```python
from build123d import *

# Parameters (mm, degrees)
F0_R     = 1.5875
F1_DEPTH = 3.048


with BuildPart() as f1:
    # F0 (on Front) → F1 (new body)
    with BuildSketch(Plane.XZ):
        with BuildLine():
            ThreePointArc((1.5875, 0), (1.122532, 1.122532), (0, 1.5875))
            ThreePointArc((0, 1.5875), (-1.122532, -1.122532), (1.5875, 0))
        make_face()
        with BuildLine():
            ThreePointArc((0.677344, -9.500886), (6.970557, -6.491299), (9.525, 0))
            ThreePointArc((9.525, 0), (6.735192, 6.735192), (0, 9.525))
            ThreePointArc((0, 9.525), (-6.534492, 6.930082), (-9.50857, 0.559208))
            ThreePointArc((-9.50857, 0.559208), (-6.930082, -6.534492), (0, -9.525))
            Line((0, -9.525), (0.677344, -9.500886))
        make_face()
        with BuildLine():
            ThreePointArc((1.5875, 0), (-1.122532, -1.122532), (0, 1.5875))
            ThreePointArc((0, 1.5875), (1.122532, 1.122532), (1.5875, 0))
        make_face(mode=Mode.SUBTRACT)
        with BuildLine():
            ThreePointArc((0, 9.525), (6.735192, 6.735192), (9.525, 0))
            ThreePointArc((9.525, 0), (6.970557, -6.491299), (0.677344, -9.500886))
            Line((0.677344, -9.500886), (44.732405, -7.932475))
            ThreePointArc((44.732405, -7.932475), (36.513756, -0.141225), (44.45, 7.9375))
            Line((44.45, 7.9375), (18.817909, 8.852932))
            ThreePointArc((18.817909, 8.852932), (13.12642, 11.553818), (11.18688, 17.547649))
            Line((11.18688, 17.547649), (15.064665, 58.492855))
            ThreePointArc((15.064665, 58.492855), (9.28782, 50.625528), (0, 47.625))
            Line((0, 47.625), (0, 9.525))
        make_face()
        with BuildLine():
            ThreePointArc((-9.50857, 0.559208), (-6.534492, 6.930082), (0, 9.525))
            Line((0, 9.525), (0, 47.625))
            ThreePointArc((0, 47.625), (-9.835501, 51.038918), (-15.440753, 59.812348))
            Line((-15.440753, 59.812348), (-9.50857, 0.559208))
        make_face()
        with BuildLine():
            ThreePointArc((0, -9.525), (0.338886, -9.51897), (0.677344, -9.500886))
            Line((0.677344, -9.500886), (0, -9.525))
        make_face()
        with BuildLine():
            Line((0, 61.9125), (0, 47.625))
            ThreePointArc((0, 47.625), (9.28782, 50.625528), (15.064665, 58.492855))
            ThreePointArc((15.064665, 58.492855), (15.671107, 60.963854), (15.875, 63.5))
            ThreePointArc((15.875, 63.5), (15.613359, 66.370305), (14.83706, 69.145998))
            ThreePointArc((14.83706, 69.145998), (9.0107, 76.569924), (0, 79.375))
            Line((0, 79.375), (0, 65.0875))
            ThreePointArc((0, 65.0875), (1.122532, 64.622532), (1.5875, 63.5))
            ThreePointArc((1.5875, 63.5), (1.122532, 62.377468), (0, 61.9125))
        make_face()
        with BuildLine():
            ThreePointArc((-15.440753, 59.812348), (-9.835501, 51.038918), (0, 47.625))
            Line((0, 47.625), (0, 61.9125))
            ThreePointArc((0, 61.9125), (-1.5875, 63.5), (0, 65.0875))
            Line((0, 65.0875), (0, 79.375))
            ThreePointArc((0, 79.375), (-9.835501, 75.961082), (-15.440753, 67.187652))
            ThreePointArc((-15.440753, 67.187652), (-15.875, 63.5), (-15.440753, 59.812348))
        make_face()
        with BuildLine():
            ThreePointArc((44.45, 7.9375), (36.513756, -0.141225), (44.732405, -7.932475))
            ThreePointArc((44.732405, -7.932475), (50.161633, -5.51191), (52.3875, 0))
            ThreePointArc((52.3875, 0), (50.06266, 5.61266), (44.45, 7.9375))
        make_face()
        with Locations((44.45, 0)):
            Circle(F0_R, mode=Mode.SUBTRACT)
        with BuildLine():
            Line((-9.452585, 115.472291), (-15.440753, 67.187652))
            ThreePointArc((-15.440753, 67.187652), (-9.835501, 75.961082), (0, 79.375))
            ThreePointArc((0, 79.375), (9.0107, 76.569924), (14.83706, 69.145998))
            Line((14.83706, 69.145998), (9.461313, 115.399625))
            ThreePointArc((9.461313, 115.399625), (9.509065, 114.850734), (9.525, 114.3))
            ThreePointArc((9.525, 114.3), (-0.587263, 104.793121), (-9.452585, 115.472291))
        make_face()
        with Locations((-2.690725, 100.0252)):
            Circle(F0_R, mode=Mode.SUBTRACT)
        with BuildLine():
            ThreePointArc((9.461313, 115.399625), (0.036594, 123.82493), (-9.452585, 115.472291))
            ThreePointArc((-9.452585, 115.472291), (-0.587263, 104.793121), (9.525, 114.3))
            ThreePointArc((9.525, 114.3), (9.509065, 114.850734), (9.461313, 115.399625))
        make_face()
        with Locations((0.111441, 114.374639)):
            Circle(F0_R, mode=Mode.SUBTRACT)
    extrude(amount=F1_DEPTH)


solid = f1.part
```
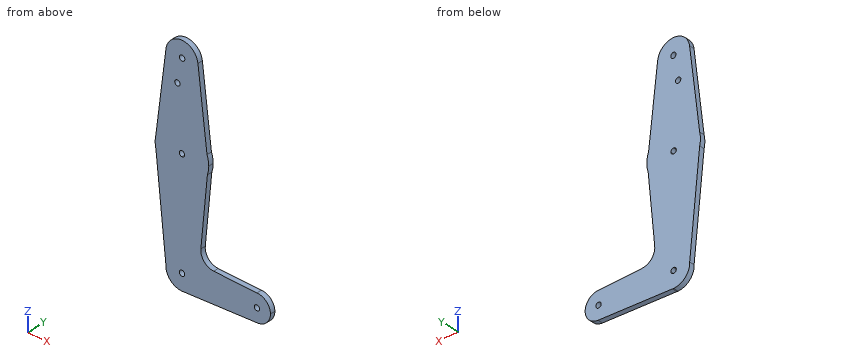
Check sheet for the modelled part. Datum: model origin and axes. Units: mm. Coordinates: 2 decimals unless noted, no trailing zeros. Write each loop counter-clockwise with the first axis right and the second up, starting at its lowest first coordinate (ties: lowest second). Pieces come first, ordered by that corner, then holes. Notation, with made-up numbers: M 14.25,52 L 19.25,52 A20 cw 19.25,74 Z; hole C -38,24.25 d3. An arc over 180 degrees is marked long. Write item = value, one per line. Start each with the question number.
1. Thickness scan on probe 1 along Z at (x, y) = (45, -0.9); probe 2 along Z at (x, y) = (43.5, -1.45); probe 3 along X at (y, z) = (-2.3, 114.5). Record the ranges inside material, lowest first.
2. Sectioned sample at D-D (x = 24). Record the cut outline in (y, z), then the cut area to 3 significant figures.
3. Sectioned sample at C-C (z = 108). Record the cut outline in (x, y), then the cut area to 3 significant figures.
4. Sectioned sample at B-B (y = -1.6). State how many separate pieces and enclosed holes the cut face has, then the cut area to 3 significant figures.
5. Go/stop test with a flat-tipped pin: pin 1 (1.5 mm diameter, centred on x = 2, y = -2, fed in from -Z). Record where the tip stops, or that it passes through.
6. Sectioned sample at A-A (x = -3). Record the cut outline in (y, z).
The answers:
q1.probe_1 = -7.92 to -1.49, 1.49 to 7.92
q1.probe_2 = -7.98 to -1.27, 1.27 to 7.97
q1.probe_3 = -9.57 to -1.47, 1.69 to 9.57
q2.outline = M -3.05,-8.67 L 0,-8.67 L 0,8.67 L -3.05,8.67 Z
q2.area = 52.8 mm²
q3.outline = M -10.38,-3.05 L 10.32,-3.05 L 10.32,0 L -10.38,0 Z
q3.area = 63.1 mm²
q4.separate_pieces = 1
q4.enclosed_holes = 5
q4.area = 3,860 mm²
q5.pin_1 = -9.48
q6.outline = M -3.05,-9.04 L 0,-9.04 L 0,98.47 L -3.05,98.47 Z; M -3.05,101.58 L 0,101.58 L 0,123.34 L -3.05,123.34 Z
